from build123d import *

# Parameters (mm, degrees)
SKETCH2_W           = 80
SKETCH2_H           = 80
SKETCH2_W_2         = 72.8
SKETCH2_H_2         = 72.8
BOSS_EXTRUDE1_DEPTH = 1042
FILLET1_R           = 1
FILLET2_R           = 1
SKETCH3_W           = 100
SKETCH3_H           = 100
BOSS_EXTRUDE2_DEPTH = 3
FILLET3_R           = 3
SKETCH5_R           = 3
CUT_EXTRUDE1_DEPTH  = 3
SKETCH6_W           = 100
SKETCH6_H           = 100
BOSS_EXTRUDE3_DEPTH = 3
FILLET4_R           = 3


with BuildPart() as part:
    # Sketch2 → Boss-Extrude1 (new body)
    with BuildSketch(Plane.XY):
        Rectangle(SKETCH2_W, SKETCH2_H)
        Rectangle(SKETCH2_W_2, SKETCH2_H_2, mode=Mode.SUBTRACT)
    extrude(amount=BOSS_EXTRUDE1_DEPTH)

    # Fillet1
    fillet1_edges = [part.edges().sort_by_distance(p)[0] for p in [
        (40, -40, 521),
        (-40, -40, 521),
        (-40, 40, 521),
        (40, 40, 521),
    ]]
    fillet(fillet1_edges, radius=FILLET1_R)

    # Fillet2
    fillet2_edges = [part.edges().sort_by_distance(p)[0] for p in [
        (-36.4, 36.4, 521),
        (-36.4, -36.4, 521),
        (36.4, -36.4, 521),
        (36.4, 36.4, 521),
    ]]
    fillet(fillet2_edges, radius=FILLET2_R)

    # Sketch3 → Boss-Extrude2 (add)
    with BuildSketch(Plane.XY.offset(1042)):
        Rectangle(SKETCH3_W, SKETCH3_H)
    extrude(amount=BOSS_EXTRUDE2_DEPTH)

    # Fillet3
    fillet3_edges = [part.edges().sort_by_distance(p)[0] for p in [
        (50, -50, 1043.5),
        (50, 50, 1043.5),
        (-50, 50, 1043.5),
        (-50, -50, 1043.5),
    ]]
    fillet(fillet3_edges, radius=FILLET3_R)

    # Sketch5 → Cut-Extrude1 (cut)
    with BuildSketch(Plane(origin=(0, 0, 1042), x_dir=(-1, 0, 0), z_dir=(0, 0, -1))):
        with Locations((15, -45)):
            Circle(SKETCH5_R)
        with Locations((-15, -45)):
            Circle(SKETCH5_R)
        with Locations((15, 45)):
            Circle(SKETCH5_R)
        with Locations((-15, 45)):
            Circle(SKETCH5_R)
    extrude(amount=-CUT_EXTRUDE1_DEPTH, mode=Mode.SUBTRACT)

    # Sketch6 → Boss-Extrude3 (add)
    with BuildSketch(Plane(origin=(0, 0, 0), x_dir=(-1, 0, 0), z_dir=(0, 0, -1))):
        Rectangle(SKETCH6_W, SKETCH6_H)
    extrude(amount=BOSS_EXTRUDE3_DEPTH)

    # Fillet4
    fillet4_edges = [part.edges().sort_by_distance(p)[0] for p in [
        (-50, -50, -1.5),
        (-50, 50, -1.5),
        (50, 50, -1.5),
        (50, -50, -1.5),
    ]]
    fillet(fillet4_edges, radius=FILLET4_R)


solid = part.part
Work out the finished part from the listing and answer in its coordinate system (mm). A direction names the side the tool comes from. Give positions to 0.01 mm unless a question says otherwise; leave off trailing zeros. Write each loop counter-clockwise with the first axis right and the second up, starting at its lowest first coordinate (ties: lowest second). Pieces come first, ordered by that corner, then holes. Notation, with made-up numbers: (-7.75, 19.25) - (-2.75, 19.25) arc R3 ccw to (-2.75, 24.25) - close; hole circle Ø4 at (0.25, 19). An arc over 180 degrees is marked (long way). One line per item, written item: value. Start each with the question number.
1. For a pull along Y with two mould halves and no side action, classify faces 1 (the flat face through (-1, -40, 514)), 2 (the flat face through (0, -36.4, 514)), 3 (the flat face through (40, -1, 514)) as +Y half, -Y half, draft (parallel to the pull), parting line (faces both ways), or undercut.
2. Given pin 1 (21 mm diameter, centred on x = 4.5, z = 447.5, fed in from -Y); pin 2 (5 mm diameter, centred on x = 23.5, z = 421, fed in from +Y); pin 3 (4 mm diameter, centred on y = -28, z = 719.5, fed in from +X), each flat-ended and moving along its own axis, determine where each tip first touches the part or whether it passes through.
3. Find section A-A (z = 894.5). Write down the section's boundary in (x, y), then the cut area to 3 significant figures.
4. Find section B-B (y = -22.5). Write down the section's boundary in (x, z), then the cut area to 3 significant figures.
5. For faces 4 (the flat face through (-1, 1, 1045)), 5 (the flat face through (-1, 40, 514)), 6 (the flat face through (1, 1, -3)), 7 (the flat face through (45, 1, 0)), 8 (the flat face through (-40, -1, 514)), determine the directions among +Z, -Z, +X, -X, +Y, -Y from which every point of the face is accessible in a straight line to the end or side of a thin tool.
6. Consider probe 1 along Y at (x, z) = (15, 1044); probe 2 along Y at (x, z) = (-7.5, 364). Determine where each line is inside the solid, lowest interval first.
Geometry results:
1. face 1: -Y half
1. face 2: undercut
1. face 3: draft
2. pin 1: y = -40
2. pin 2: y = 40
2. pin 3: x = 40
3. outline: (-40, -39) arc R1 ccw to (-39, -40) - (39, -40) arc R1 ccw to (40, -39) - (40, 39) arc R1 ccw to (39, 40) - (-39, 40) arc R1 ccw to (-40, 39) - close; hole (-36.4, -35.4) arc R1 ccw to (-35.4, -36.4) - (35.4, -36.4) arc R1 ccw to (36.4, -35.4) - (36.4, 35.4) arc R1 ccw to (35.4, 36.4) - (-35.4, 36.4) arc R1 ccw to (-36.4, 35.4) - close
3. area: 1,100 mm2
4. outline: (-50, -3) - (50, -3) - (50, 0) - (40, 0) - (40, 1042) - (50, 1042) - (50, 1045) - (-50, 1045) - (-50, 1042) - (-40, 1042) - (-40, 0) - (-50, 0) - close; hole (-36.4, 0) - (36.4, 0) - (36.4, 1042) - (-36.4, 1042) - close
4. area: 8,100 mm2
5. face 4: +Z, +X, -X, +Y, -Y
5. face 5: +X, -X, +Y
5. face 6: -Z, +X, -X, +Y, -Y
5. face 7: none
5. face 8: -X, +Y, -Y
6. probe 1: -50 to -48, -42 to 42, 48 to 50
6. probe 2: -40 to -36.4, 36.4 to 40
